Part model, mm, in its own coordinate system. Face numbers are marked on the shaded views. A direction names the side the tool comes from. Round coordinates to 2 decimals unless told otherwise and drop trailing zeros. Loops run counter-clockwise (first coordinate to the right, second up) from the corner with the lowest first, then second, coordinate; pieces in that order, holes last. Notation, with made-up numbers: (35.5, 53) -> (69.5, 53) arc R30 cw to (69.5, 88) -> close; hole circle Ø10 at (61.5, 88). An arc over 180 degrees is marked (long way). Use a Markdown table: item, result. Add a question column.
Item 1: Cut at B-B, the plane y = 12. List the corners of the cut face in (x, z).
Item 2: Two-plate mould, pull along Y, no slides. Class the marked faces 1, 2 and 3: pulls with the +Y half, pulls with the -Y half, needs draft (parallel to the pull), parting line crosses it, or undercut.
Item 3: Cut at A-A, the plane z = -11. List the corners of the cut face in (x, y).
Item 4: Probe line 1 (Z direction, x = 9.25, y = 1.5); line 2 (X direction, y = 9, z = 3); line 3 (Y direction, x = -7, z = -9.25). List the from-to ranges inside material, lowest first. Write a range as [from, to].
Item 5: Cut at C-C, the plane x = -2.5. List the corners of the cut face in (y, z), plus the area to 3 significant figures.
Item 6: Flat gauge pins, fed straight in: pin 1 (0.6 mm diameter, centred on x = 0.5, y = 1, fed in from -Z); pin 2 (6 mm diameter, centred on x = -2, z = 10, fed in from +Y); pin 3 (12 mm diameter, centred on x = 0, z = -7.5, fed in from +Y). Where does each tip first touch, or does it go through?
Item 7: Cut at D-D, the plane z = 3.5. List the corners of the cut face in (x, y), plus the area to 3 significant figures.
Item 8: Which spindle directions (+Z, -Z, +X, -X, +Y, -Y) get a long thin tool onto all of the face, cutting with end or side? Do the marked faces 4, 5 and 6. Say none if no direction does.
```python
from build123d import *

# Parameters (mm, degrees)
SKETCH1_W           = 25
SKETCH1_H           = 25
BOSS_EXTRUDE1_DEPTH = 2.5
SKETCH2_R           = 5.5
BOSS_EXTRUDE2_DEPTH = 2
SKETCH3_W           = 3
SKETCH3_H           = 10.583005244
BOSS_EXTRUDE3_DEPTH = 12
CUT_EXTRUDE1_DEPTH  = 15
SKETCH6_W           = 2
SKETCH6_H           = 8
SKETCH6_W_2         = 8
SKETCH6_H_2         = 2
CUT_EXTRUDE2_DEPTH  = 15
SKETCH7_R           = 0.75
CUT_EXTRUDE3_DEPTH  = 10


with BuildPart() as part:
    # Sketch1 → Boss-Extrude1 (new body)
    with BuildSketch(Plane(origin=(0, 0, 0), x_dir=(1, 0, 0), z_dir=(0, 1, 0))):
        Rectangle(SKETCH1_W, SKETCH1_H)
    extrude(amount=BOSS_EXTRUDE1_DEPTH)

    # Sketch2 → Boss-Extrude2 (add)
    with BuildSketch(Plane(origin=(0, 2.5, 0), x_dir=(1, 0, 0), z_dir=(0, 1, 0))):
        with Locations(Location((0, 0, 0), (0, 0, 270))):
            Circle(SKETCH2_R)
    extrude(amount=BOSS_EXTRUDE2_DEPTH)

    # Sketch3 → Boss-Extrude3 (add)
    with BuildSketch(Plane(origin=(0, 4.5, 0), x_dir=(1, 0, 0), z_dir=(0, 1, 0))):
        with BuildLine():
            ThreePointArc((1.5, 5.291502622), (0, 5.5), (-1.5, 5.291502622))
            Line((-1.5, 5.291502622), (1.5, 5.291502622))
        make_face()
        Rectangle(SKETCH3_W, SKETCH3_H)
        with BuildLine():
            Line((1.5, -5.291502622), (-1.5, -5.291502622))
            ThreePointArc((-1.5, -5.291502622), (0, -5.5), (1.5, -5.291502622))
        make_face()
    extrude(amount=BOSS_EXTRUDE3_DEPTH)

    # Sketch4 → Cut-Extrude1 (cut)
    with BuildSketch(Plane(origin=(1.5, 0, 0), x_dir=(0, 0, -1), z_dir=(1, 0, 0))):
        with BuildLine():
            Line((-5.5, 17.101407095), (-5.5, 11))
            ThreePointArc((-5.5, 11), (-5.447626291, 11.757210532), (-5.291502622, 12.5))
            Line((-5.291502622, 12.5), (-5.291502622, 16.5))
            Line((-5.291502622, 16.5), (0, 16.5))
            Line((0, 16.5), (5.291502622, 16.5))
            Line((5.291502622, 16.5), (5.291502622, 12.5))
            ThreePointArc((5.291502622, 12.5), (5.447626291, 11.757210532), (5.5, 11))
            Line((5.5, 11), (5.5, 17.101407095))
            Line((5.5, 17.101407095), (-5.5, 17.101407095))
        make_face()
        with BuildLine():
            Line((-5.291502622, 16.5), (-5.291502622, 12.5))
            ThreePointArc((-5.291502622, 12.5), (-3.31662479, 15.387482194), (0, 16.5))
            Line((0, 16.5), (-5.291502622, 16.5))
        make_face()
        with BuildLine():
            Line((5.291502622, 16.5), (0, 16.5))
            ThreePointArc((0, 16.5), (3.31662479, 15.387482194), (5.291502622, 12.5))
            Line((5.291502622, 12.5), (5.291502622, 16.5))
        make_face()
    extrude(amount=-CUT_EXTRUDE1_DEPTH, mode=Mode.SUBTRACT)

    # Sketch6 → Cut-Extrude2 (cut)
    with BuildSketch(Plane(origin=(0, 2.5, 0), x_dir=(1, 0, 0), z_dir=(0, 1, 0))):
        with Locations((0, 12.5)):
            Rectangle(SKETCH6_W, SKETCH6_H)
        with Locations((0, -12.5)):
            Rectangle(SKETCH6_W, SKETCH6_H)
        with Locations((12.5, 0)):
            Rectangle(SKETCH6_W_2, SKETCH6_H_2)
        with Locations((-12.5, 0)):
            Rectangle(SKETCH6_W_2, SKETCH6_H_2)
    extrude(amount=-CUT_EXTRUDE2_DEPTH, mode=Mode.SUBTRACT)

    # Sketch7 → Cut-Extrude3 (cut)
    with BuildSketch(Plane(origin=(1.5, 0, 0), x_dir=(0, 0, -1), z_dir=(1, 0, 0))):
        with Locations((0, 12)):
            Circle(SKETCH7_R)
    extrude(amount=-CUT_EXTRUDE3_DEPTH, mode=Mode.SUBTRACT)


solid = part.part
```
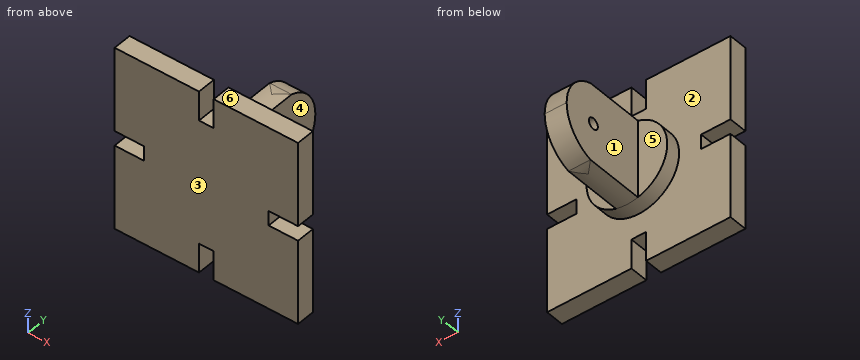
A:
| question | item | result |
|---|---|---|
| 1 | outline | (-1.5, -5.29) arc R5.5 ccw to (-1, -5.41) -> (1, -5.41) arc R5.5 ccw to (1.5, -5.29) -> (1.5, -0.75) -> (-1.5, -0.75) -> close; (-1.5, 0.75) -> (1.5, 0.75) -> (1.5, 5.29) arc R5.5 ccw to (1, 5.41) -> (-1, 5.41) arc R5.5 ccw to (-1.5, 5.29) -> close |
| 2 | face 1 | needs draft |
| 2 | face 2 | pulls with the +Y half |
| 2 | face 3 | pulls with the -Y half |
| 3 | outline | (-12.5, 0) -> (-1, 0) -> (-1, 2.5) -> (-12.5, 2.5) -> close; (1, 0) -> (12.5, 0) -> (12.5, 2.5) -> (1, 2.5) -> close |
| 4 | line 1 | z = [-12.5, -1], [1, 12.5] |
| 4 | line 2 | x = [-1.5, 1.5] |
| 4 | line 3 | y = [0, 2.5] |
| 5 | outline | (0, -12.5) -> (2.5, -12.5) -> (2.5, -4.9) -> (4.5, -4.9) -> (4.5, 4.9) -> (2.5, 4.9) -> (2.5, 12.5) -> (0, 12.5) -> close |
| 5 | area | 82.1 mm^2 |
| 6 | pin 1 | stops at z = -8.5 |
| 6 | pin 2 | stops at y = 2.5 |
| 6 | pin 3 | stops at y = 16.29 |
| 7 | outline | (-12.5, 0) -> (12.5, 0) -> (12.5, 2.5) -> (4.24, 2.5) -> (4.24, 4.5) -> (1.5, 4.5) -> (1.5, 15.24) -> (-1.5, 15.24) -> (-1.5, 4.5) -> (-4.24, 4.5) -> (-4.24, 2.5) -> (-12.5, 2.5) -> close |
| 7 | area | 112 mm^2 |
| 8 | face 4 | +Z, -Z, +X, +Y |
| 8 | face 5 | +Z, -Z, -X, +Y |
| 8 | face 6 | +Z, +X, -X, +Y, -Y |
